For this review, take the finished solid that the model builds, in its own axes (mm). A direction names the side the tool comes from. Round coordinates to 2 decimals unless told otherwise and drop trailing zeros. Order: outer loops, then holes, each group sorted by start corner. A loop starts at its lowest first (then second) coordinate and runs counter-clockwise, first axis right, second up. Notation, with made-up numbers: M 31.5,36.5 L 44.5,36.5 A15 ccw 44.5,49.5 Z; hole C -8.5,42 d1. An arc over 180 degrees is marked long. Use a Markdown table: item, result.
from build123d import *

# Parameters (mm, degrees)
F1_DEPTH = 9
F2_DEPTH = 6
F3_DEPTH = 7


with BuildPart() as f1:
    # F0 (on Right) → F1 (new body)
    with BuildSketch(Plane.YZ):
        with BuildLine():
            Line((0, 115), (-67.5, 115))
            Line((-67.5, 115), (-67.5, -115))
            Line((-67.5, -115), (0, -115))
            Line((0, -115), (0, -97.5))
            Line((0, -97.5), (-50, -97.5))
            Line((-50, -97.5), (-50, 30.4482906163))
            Line((-50, 30.4482906163), (-50, 39.5))
            Line((-50, 39.5), (0, 39.5))
            Line((0, 39.5), (0, 51))
            ThreePointArc((0, 51), (-22, 73), (0, 95))
            Line((0, 95), (0, 115))
        make_face()
        with BuildLine():
            Line((67.5, 115), (0, 115))
            Line((0, 115), (0, 95))
            ThreePointArc((0, 95), (15.5563491861, 88.5563491861), (22, 73))
            ThreePointArc((22, 73), (15.5563491861, 57.4436508139), (0, 51))
            Line((0, 51), (0, 39.5))
            Line((0, 39.5), (50, 39.5))
            Line((50, 39.5), (50, 30.4482906163))
            Line((50, 30.4482906163), (50, -97.5))
            Line((50, -97.5), (0, -97.5))
            Line((0, -97.5), (0, -115))
            Line((0, -115), (67.5, -115))
            Line((67.5, -115), (67.5, 115))
        make_face()
    extrude(amount=F1_DEPTH)

    # F0 (on Right) → F2 (join)
    with BuildSketch(Plane.YZ):
        with BuildLine():
            Line((0, 89.5), (0, 95))
            ThreePointArc((0, 95), (-22, 73), (0, 51))
            Line((0, 51), (0, 56.5))
            ThreePointArc((0, 56.5), (-16.5, 73), (0, 89.5))
        make_face()
        with BuildLine():
            ThreePointArc((22, 73), (15.5563491861, 88.5563491861), (0, 95))
            Line((0, 95), (0, 89.5))
            ThreePointArc((0, 89.5), (11.6672618896, 84.6672618896), (16.5, 73))
            ThreePointArc((16.5, 73), (11.6672618896, 61.3327381104), (0, 56.5))
            Line((0, 56.5), (0, 51))
            ThreePointArc((0, 51), (15.5563491861, 57.4436508139), (22, 73))
        make_face()
    extrude(amount=F2_DEPTH)

    # F0 (on Right) → F3 (join)
    with BuildSketch(Plane.YZ):
        Polygon((-50, -97.5), (0, -97.5), (0, -76.5), (-37.5, -76.5), (-37.5, 18.5), (0, 18.5), (0, 39.5), (-50, 39.5), (-50, 30.4482906163), align=None)
        Polygon((0, -76.5), (0, -97.5), (50, -97.5), (50, 30.4482906163), (50, 39.5), (0, 39.5), (0, 18.5), (37.5, 18.5), (37.5, -76.5), align=None)
    extrude(amount=F3_DEPTH)


solid = f1.part
Q1. Add section A-A (x = 4.5). Write out the cut boundary in (y, z).
Determined:
| item | result |
|---|---|
| outline | M -67.5,-115 L 67.5,-115 L 67.5,115 L -67.5,115 Z; hole M -37.5,-76.5 L 37.5,-76.5 L 37.5,18.5 L -37.5,18.5 Z; hole C 0,73 d33 |
Q2. Wall thickness on line 1 along Z through (x, y) = (8.45, 0); line 2 along Y through (x, z) = (4.5, 1.5); line 3 along Y through (x, z) = (6.7, 73): over which ranges is each line inside the solid? List them lowest first. Write a range as [from, to].
Determined:
| item | result |
|---|---|
| line 1 | z = [-115, -97.5], [39.5, 51], [95, 115] |
| line 2 | y = [-67.5, -37.5], [37.5, 67.5] |
| line 3 | y = [-67.5, -22], [22, 67.5] |
Q3. Add section C-C (z = -8). Write out the cut boundary in (x, y).
Determined:
| item | result |
|---|---|
| outline | M 0,-67.5 L 9,-67.5 L 9,-50 L 7,-50 L 7,-37.5 L 0,-37.5 Z; M 0,37.5 L 7,37.5 L 7,50 L 9,50 L 9,67.5 L 0,67.5 Z |
Q4. Machinability: for faces 1 (the flat face through (3, -37.5, -30)), 2 (the flat face through (7, 44, -28)), 3 (the flat face through (0, -1, 27)), which of the approach directions +Z, -Z, +X, -X, +Y, -Y give a long, thin tool a straight path to every point of the face, cutting with its end or side? Answer none if there is none.
Determined:
| item | result |
|---|---|
| face 1 | +X, -X |
| face 2 | +X |
| face 3 | +Z, -Z, -X, +Y, -Y |
Q5. Add section D-D (y = 45). Write out the cut boundary in (x, z).
Determined:
| item | result |
|---|---|
| outline | M 0,-115 L 9,-115 L 9,-97.5 L 7,-97.5 L 7,39.5 L 9,39.5 L 9,115 L 0,115 Z |
Q6. Add section B-B (y = 30). Write out the cut boundary in (x, z), then the cut area to 3 significant figures.
Determined:
| item | result |
|---|---|
| outline | M 0,-115 L 9,-115 L 9,-97.5 L 7,-97.5 L 7,-76.5 L 0,-76.5 Z; M 0,18.5 L 7,18.5 L 7,39.5 L 9,39.5 L 9,115 L 0,115 Z |
| area | 1,130 mm^2 |
Q7. Draft analysis for pull direction Y (two halves, no side actions). For faces 4 (the flat face through (4, -67.5, 2)), 5 (the flat face through (6, 3.2, 89.4)), 6 (the flat face through (4, 1, 115)), 7 (the flat face through (4, 67.5, -2)), state which applies: pulls with the +Y half, pulls with the -Y half, needs draft (parallel to the pull), parting line crosses it, or undercut.
Determined:
| item | result |
|---|---|
| face 4 | pulls with the -Y half |
| face 5 | undercut |
| face 6 | needs draft |
| face 7 | pulls with the +Y half |
Q8. Clearance check with a flat-ended pin moving along its axis: pin 1 (13 mm diameter, centred on y = -3.5, z = 67.5, fed in from +X). State where the tip first meets the part, or that it passes through.
Determined:
| item | result |
|---|---|
| pin 1 | passes through |
